Geometry: final body of the model. Coordinates: model frame, mm. A direction names the side the tool comes from. Give positions to 0.01 mm unless a question says otherwise; leave off trailing zeros. Order: outer loops, then holes, each group sorted by start corner. A loop starts at its lowest first (then second) coordinate and runs counter-clockwise, first axis right, second up. Notation, with made-up numbers: (-11, 78.5) -> (43, 78.5) arc R17 ccw to (43, 105.5) -> close; hole circle Ø8 at (38.5, 48). An arc over 180 degrees is marked (long way). Write item = value, one per line.
```python
from build123d import *

# Parameters (mm, degrees)
SKETCH_1_R      = 2.3
EXTRUDE_1_DEPTH = 5.2


with BuildPart() as part:
    # 草图1 → 凸台-拉伸1 (new body)
    with BuildSketch(Plane.XY):
        with BuildLine():
            Line((-5, 13), (-5, 0))
            ThreePointArc((-5, 0), (-3.535533906, -3.535533906), (0, -5))
            Line((0, -5), (25, -5))
            ThreePointArc((25, -5), (28.535533906, -3.535533906), (30, 0))
            Line((30, 0), (30, 13))
            ThreePointArc((30, 13), (28.535533906, 16.535533906), (25, 18))
            Line((25, 18), (0, 18))
            ThreePointArc((0, 18), (-3.535533906, 16.535533906), (-5, 13))
        make_face()
        with Locations((0, 13)):
            Circle(SKETCH_1_R, mode=Mode.SUBTRACT)
        with Locations((25, 13)):
            Circle(SKETCH_1_R, mode=Mode.SUBTRACT)
        Circle(SKETCH_1_R, mode=Mode.SUBTRACT)
        with Locations((25, 0)):
            Circle(SKETCH_1_R, mode=Mode.SUBTRACT)
        with BuildLine():
            Line((5, 13), (20, 13))
            ThreePointArc((20, 13), (20.816699867, 10.261387212), (23, 8.417424305))
            Line((23, 8.417424305), (23, 4.582575695))
            ThreePointArc((23, 4.582575695), (20.816699867, 2.738612788), (20, 0))
            Line((20, 0), (5, 0))
            ThreePointArc((5, 0), (4.183300133, 2.738612788), (2, 4.582575695))
            Line((2, 4.582575695), (2, 8.417424305))
            ThreePointArc((2, 8.417424305), (4.183300133, 10.261387212), (5, 13))
        make_face(mode=Mode.SUBTRACT)
    extrude(amount=EXTRUDE_1_DEPTH)


solid = part.part
```
1) Reachability of faces 1 (the face through (2, 6, 3)), 2 (the face through (-5, 7, 3)) from +Z, -Z, +X, -X, +Y, -Y: full face, straight path, thin tool, end or side. Return the list, or none.
Check sheet entries:
face_1 = +Z, -Z
face_2 = +Z, -Z, -X, +Y, -Y
2) Section query A-A (x = 22). Output: boundary loops of the cut face in (y, z), plus the area to 3 significant figures.
Check sheet entries:
outline = (-5, 0) -> (4, 0) -> (4, 5.2) -> (-5, 5.2) -> close; (9, 0) -> (18, 0) -> (18, 5.2) -> (9, 5.2) -> close
area = 93.6 mm²
3) Mould query, pull axis X, two halves, no side actions, for faces 3 (the face through (4, 10, 3)), 4 (the face through (-4, -3, 3)), 5 (the face through (30, 6, 3)), 6 (the face through (12, -1, 0)). Classes: +X half, -X half, draft (parallel to the pull), parting line (faces both ways), or undercut.
Check sheet entries:
face_3 = undercut
face_4 = -X half
face_5 = +X half
face_6 = draft
4) Section query C-C (z = 4.3). Output: boundary loops of the cut face in (x, y).
Check sheet entries:
outline = (-5, 0) arc R5 ccw to (0, -5) -> (25, -5) arc R5 ccw to (30, 0) -> (30, 13) arc R5 ccw to (25, 18) -> (0, 18) arc R5 ccw to (-5, 13) -> close; hole circle Ø4.6 at (0, 0); hole circle Ø4.6 at (0, 13); hole (2, 4.58) arc R5 cw to (5, 0) -> (20, 0) arc R5 cw to (23, 4.58) -> (23, 8.42) arc R5 cw to (20, 13) -> (5, 13) arc R5 cw to (2, 8.42) -> close; hole circle Ø4.6 at (25, 0); hole circle Ø4.6 at (25, 13)
5) Line query: line 1 (Y direction, x = 25, z = 3.2); line 2 (Y direction, x = 19.5, z = 3.6); line 3 (X direction, y = 14, z = 2.15). Output: solid intervals per line, ascending. Write a range as from..to.
Check sheet entries:
line_1 = -5..-2.3, 2.3..10.7, 15.3..18
line_2 = -5..0, 13..18
line_3 = -4.9..-2.07, 2.07..22.93, 27.07..29.9
6) Section query B-B (y = 3). Output: boundary loops of the cut face in (x, z), plus the area to 3 significant figures.
Check sheet entries:
outline = (-5, 0) -> (4, 0) -> (4, 5.2) -> (-5, 5.2) -> close; (21, 0) -> (30, 0) -> (30, 5.2) -> (21, 5.2) -> close
area = 93.6 mm²
